Autodesk Inventor part; units mm, degrees
ref_plane "YZ Plane" through (0, 0, 0) normal (1, 0, 0) x (0, 1, 0)
ref_plane "XZ Plane" through (0, 0, 0) normal (0, 1, 0) x (-1, 0, 0)
ref_plane "XY Plane" through (0, 0, 0) normal (0, 0, 1) x (1, 0, 0)
sketch "Sketch1" plane through (0, 0, 0) normal (0, 1, 0) x (-1, 0, 0)
  circle A0 centre (0, 0) radius 21.5
  circle A1 centre (0, 0) radius 30
  dimension "d0" = 43
  dimension "d1" = 60
extrude "Extrusion1" add sketch "Sketch1" along normal blind 5
sketch "Sketch2" plane through (0, 5, 0) normal (0, 1, 0) x (1, 0, 0)
  line L0 (18.5, -18.5) -> (-18.5, -18.5)
  line L1 (-18.5, -18.5) -> (-18.5, 18.5)
  line L2 (-18.5, 18.5) -> (18.5, 18.5)
  line L3 (18.5, 18.5) -> (18.5, -18.5)
  circle A0 centre (0, 0) radius 30
  line L4 (18.5, -18.5) -> (-18.5, 18.5) construction
  line L5 (-18.5, -18.5) -> (18.5, 18.5) construction
  dimension "d4" = 37
  dimension "d5" = 37
hole "Hole1" at (-18.5, 5, 18.5) at (-18.5, 5, -18.5) at (18.5, 5, -18.5) at (18.5, 5, 18.5) direction (0, -1, 0) diameter 4.496 depth 6
properties part number "immersion_chamber_plate"
Read the model definition and answer for the solid it produces. Units are mm, in the model's axes. Coordinates: 2 decimals unless noted, no trailing zeros. Loops run counter-clockwise (first coordinate to the right, second up) from the corner with the lowest first, then second, coordinate; pieces in that order, holes last. Notation, with made-up numbers: (78.5, -10) -> (128.5, -10) arc R33 ccw to (128.5, 28) -> close; hole circle Ø5 at (84.5, 63). An arc over 180 degrees is marked (long way). Return JSON: item names as keys, results as strings.
Item 1: Find section D-D (z = 18.5). Determine the outline of the cut face in (x, y).
Answers:
{"outline": "(-23.62, 0) -> (-20.75, 0) -> (-20.75, 5) -> (-23.62, 5) -> close; (-16.25, 0) -> (-10.95, 0) -> (-10.95, 5) -> (-16.25, 5) -> close; (10.95, 0) -> (16.25, 0) -> (16.25, 5) -> (10.95, 5) -> close; (20.75, 0) -> (23.62, 0) -> (23.62, 5) -> (20.75, 5) -> close"}
Item 2: Find section A-A (z = 0). Determine the outline of the cut face in (x, y), plus the area to 3 significant figures.
Answers:
{"outline": "(-30, 0) -> (-21.5, 0) -> (-21.5, 5) -> (-30, 5) -> close; (21.5, 0) -> (30, 0) -> (30, 5) -> (21.5, 5) -> close", "area": "85.0 mm2"}
Item 3: Find section B-B (x = -18.5). Determine the outline of the cut face in (y, z), plus the area to 3 significant figures.
Answers:
{"outline": "(0, -23.62) -> (5, -23.62) -> (5, -20.75) -> (0, -20.75) -> close; (0, -16.25) -> (5, -16.25) -> (5, -10.95) -> (0, -10.95) -> close; (0, 10.95) -> (5, 10.95) -> (5, 16.25) -> (0, 16.25) -> close; (0, 20.75) -> (5, 20.75) -> (5, 23.62) -> (0, 23.62) -> close", "area": "81.7 mm2"}
Item 4: Flat-ended cylindrical pins translate along their axes: P1, Ø3, axis at x = -7.5, y = 2, coming from the -Z side; P2, Ø3, axis at y = 0.5, z = -22, coming from the -X side. Find the tip coordinate at first contact, or state that the pin passes through.
Answers:
{"P1": "stops at z = -29.39", "P2": "stops at x = -21.9"}
Item 5: For a pull along X with two mould halves and no side action, classify faces 1 (the flat face through (-15.4, 0, -15.4)), 2 (the cylindrical face through (16.6, 2.5, 19.7)), 3 (the cylindrical face through (29.97, 2.46, -1.32)), 4 (the cylindrical face through (2.799, 2.465, -21.317)) as +X half, -X half, draft (parallel to the pull), parting line (faces both ways), or undercut.
Answers:
{"face 1": "draft", "face 2": "undercut", "face 3": "parting line", "face 4": "undercut"}
Item 6: Find section C-C (x = 0). Determine the outline of the cut face in (y, z).
Answers:
{"outline": "(0, -30) -> (5, -30) -> (5, -21.5) -> (0, -21.5) -> close; (0, 21.5) -> (5, 21.5) -> (5, 30) -> (0, 30) -> close"}
Item 7: Find the intervals of material crossed by probe 1 along Z at (x, y) = (0, 4.05); probe 2 along X at (y, z) = (2.7, -18.5), in increasing order.
Answers:
{"probe 1": "z = -30 to -21.5, 21.5 to 30", "probe 2": "x = -23.62 to -20.75, -16.25 to -10.95, 10.95 to 16.25, 20.75 to 23.62"}
